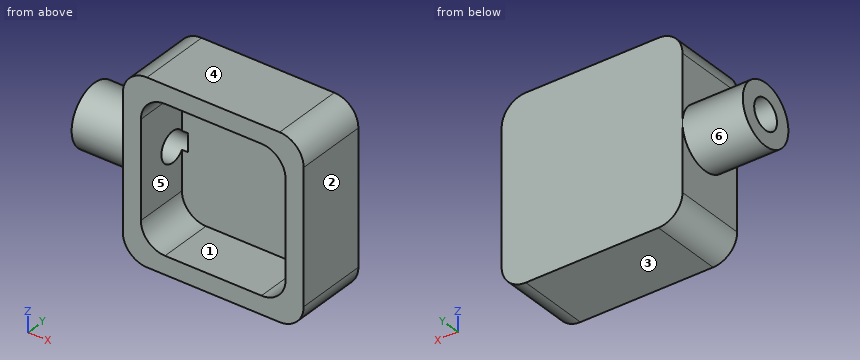
from build123d import *

# Parameters (mm, degrees)
F1_DEPTH = 1.5
F2_DEPTH = 6
F3_R     = 1.25
F4_DEPTH = 2
F5_DEPTH = 5


with BuildPart() as f1:
    # F0 (on Front) → F1 (new body)
    with BuildSketch(Plane.XZ):
        with BuildLine():
            Line((-4, -6), (4, -6))
            ThreePointArc((4, -6), (5.414214, -5.414214), (6, -4))
            Line((6, -4), (6, 4))
            ThreePointArc((6, 4), (5.414214, 5.414214), (4, 6))
            Line((4, 6), (-4, 6))
            ThreePointArc((-4, 6), (-5.414214, 5.414214), (-6, 4))
            Line((-6, 4), (-6, -4))
            ThreePointArc((-6, -4), (-5.414214, -5.414214), (-4, -6))
        make_face()
    extrude(amount=F1_DEPTH)

    # F0 (on Front) → F2 (join)
    with BuildSketch(Plane.XZ):
        with BuildLine():
            Line((-5.5, -7.5), (5.5, -7.5))
            ThreePointArc((5.5, -7.5), (6.914214, -6.914214), (7.5, -5.5))
            Line((7.5, -5.5), (7.5, 5.5))
            ThreePointArc((7.5, 5.5), (6.914214, 6.914214), (5.5, 7.5))
            Line((5.5, 7.5), (-5.5, 7.5))
            ThreePointArc((-5.5, 7.5), (-6.914214, 6.914214), (-7.5, 5.5))
            Line((-7.5, 5.5), (-7.5, -5.5))
            ThreePointArc((-7.5, -5.5), (-6.914214, -6.914214), (-5.5, -7.5))
        make_face()
        with BuildLine():
            ThreePointArc((6, -4), (5.414214, -5.414214), (4, -6))
            Line((4, -6), (-4, -6))
            ThreePointArc((-4, -6), (-5.414214, -5.414214), (-6, -4))
            Line((-6, -4), (-6, 4))
            ThreePointArc((-6, 4), (-5.414214, 5.414214), (-4, 6))
            Line((-4, 6), (4, 6))
            ThreePointArc((4, 6), (5.414214, 5.414214), (6, 4))
            Line((6, 4), (6, -4))
        make_face(mode=Mode.SUBTRACT)
    extrude(amount=F2_DEPTH)

    # F3 (on face) → F4 (cut)
    with BuildSketch(Plane(origin=(-7.5, 0, 0), x_dir=(0, -1, 0), z_dir=(-1, 0, 0))):
        with Locations((2.5, 0)):
            Circle(F3_R)
    extrude(amount=-F4_DEPTH, mode=Mode.SUBTRACT)

    # F3 (on face) → F5 (join)
    with BuildSketch(Plane(origin=(-7.5, 0, 0), x_dir=(0, -1, 0), z_dir=(-1, 0, 0))):
        with BuildLine():
            ThreePointArc((0, 0), (2.5, -2.5), (5, 0))
            ThreePointArc((5, 0), (2.5, 2.5), (0, 0))
        make_face()
        with Locations((2.5, 0)):
            Circle(F3_R, mode=Mode.SUBTRACT)
    extrude(amount=F5_DEPTH)


solid = f1.part
Geometry check sheet. Reference: the model listing, model coordinates, mm. Face numbers are marked on the shaded views. A direction names the side the tool comes from. Round coordinates to 2 decimals unless told otherwise and drop trailing zeros. Order: outer loops, then holes, each group sorted by start corner. A loop starts at its lowest first (then second) coordinate and runs counter-clockwise, first axis right, second up. Notation, with made-up numbers: M 85,53.25 L 95,53.25 A32 cw 95,89.25 Z; hole C 56.25,57 d1. An arc over 180 degrees is marked long. Answer in a Markdown table with one row per item. Add a question column.
Item 1: Sectioned sample at C-C, the plane z = 2. Enter the section's corners in (x, y), plus the area to 3 significant figures.
Item 2: Draft check along Z on the marked faces 1, 2 and 3. Enter one of: released by +Z, released by -Z, zero draft, split by the parting line, or undercut.
Item 3: Set-up check for the marked faces 4, 5 and 6: record each of +Z, -Z, +X, -X, +Y, -Y from which the full face is reachable in a straight line by a thin tool's end or side.
Item 4: Material ranges on L1, parallel to Z at x = -8.6, y = -2.5; L2, parallel to Y at x = -6.4, z = 0; L3, parallel to X at y = -1.75, z = 4, recorded low to high. Write a range as [from, to].
Item 5: Sectioned sample at A-A, the plane y = -4.5. Enter the section's corners in (x, z).
Item 6: Depth check by flat-ended pin: pin 1 Ø1.5 at (y, z) = (-1, -4.5) entering from -X; pin 2 Ø3 at (x, z) = (-10.5, -2.5) entering from -Y; pin 3 Ø3 at (y, z) = (-3.5, 0) entering from -X; pin 4 Ø4 at (x, z) = (0.5, -2.5) entering from -Y. Enter the tip coordinate at first touch or a pass-through.
Item 7: Sectioned sample at B-B, the plane x = 2.5. Enter the section's corners in (y, z), plus the area to 3 significant figures.
Item 8: Sectioned sample at D-D, the plane y = -2.5. Enter the section's corners in (x, z).
Filled in:
| question | item | result |
|---|---|---|
| 1 | outline | M -12.5,-4 L -7.5,-4 L -7.5,-6 L -6,-6 L -6,-1.5 L 6,-1.5 L 6,-6 L 7.5,-6 L 7.5,0 L -7.5,0 L -7.5,-1 L -12.5,-1 Z |
| 1 | area | 51.0 mm² |
| 2 | face 1 | undercut |
| 2 | face 2 | zero draft |
| 2 | face 3 | released by -Z |
| 3 | face 4 | +Z, +X, -X, +Y, -Y |
| 3 | face 5 | -Y |
| 3 | face 6 | -X |
| 4 | L1 | z = [-2.5, -1.25], [1.25, 2.5] |
| 4 | L2 | y = [-6, -3.75], [-1.25, 0] |
| 4 | L3 | x = [-7.5, -6], [6, 7.5] |
| 5 | outline | M -12.5,-1.5 L -7.5,-1.5 L -7.5,-5.5 A2 ccw -5.5,-7.5 L 5.5,-7.5 A2 ccw 7.5,-5.5 L 7.5,5.5 A2 ccw 5.5,7.5 L -5.5,7.5 A2 ccw -7.5,5.5 L -7.5,1.5 L -12.5,1.5 Z; hole M -6,-4 A2 ccw -4,-6 L 4,-6 A2 ccw 6,-4 L 6,4 A2 ccw 4,6 L -4,6 A2 ccw -6,4 Z |
| 6 | pin 1 | stops at x = -7.5 |
| 6 | pin 2 | stops at y = -4.79 |
| 6 | pin 3 | stops at x = -12.5 |
| 6 | pin 4 | stops at y = -1.5 |
| 7 | outline | M -6,-7.5 L 0,-7.5 L 0,7.5 L -6,7.5 L -6,6 L -1.5,6 L -1.5,-6 L -6,-6 Z |
| 7 | area | 36.0 mm² |
| 8 | outline | M -12.5,-2.5 L -7.5,-2.5 L -7.5,-5.5 A2 ccw -5.5,-7.5 L 5.5,-7.5 A2 ccw 7.5,-5.5 L 7.5,5.5 A2 ccw 5.5,7.5 L -5.5,7.5 A2 ccw -7.5,5.5 L -7.5,2.5 L -12.5,2.5 L -12.5,1.25 L -6,1.25 L -6,4 A2 cw -4,6 L 4,6 A2 cw 6,4 L 6,-4 A2 cw 4,-6 L -4,-6 A2 cw -6,-4 L -6,-1.25 L -12.5,-1.25 Z |
